Model file for the job. Use its own axes, mm. A direction names the side the tool comes from. Round coordinates to 2 decimals unless told otherwise and drop trailing zeros. Order: outer loops, then holes, each group sorted by start corner. A loop starts at its lowest first (then second) coordinate and runs counter-clockwise, first axis right, second up. Notation, with made-up numbers: (-34.5, 17.5) -> (9.5, 17.5) arc R9 ccw to (9.5, 30.5) -> close; hole circle Ø3 at (-17, 43.25). An arc over 180 degrees is marked (long way). Put each result on its own line as item: value. Start each with the question number.
Q1. 3-axis set-ups, long thin cutter, end or side, ignore diameter. For faces 5 (the face through (-48, 44, 2)), 6 (the face through (30, 44, 2)), 7 (the face through (40, -40, 2)): which of +Z, -Z, +X, -X, +Y, -Y reach the whole face in a straight line?
Q2. Flat gauge pins, fed straight in: P1, Ø1.2, axis at y = -41.5, z = 1, coming from the +X side; P2, Ø1.2, axis at y = -42, z = 2.5, coming from the -X side; P3, Ø2, axis at x = -1, z = 2.5, coming from the +Y side; P4, Ø3, axis at x = 24, y = -5.5, coming from the -Z side. Where does each tip first touch, or does it go through?
Q3. Cut at A-A, the plane y = 41.5. List the corners of the cut face in (x, z).
Q4. Pull direction X, two halves, no side cores. Call faces 1 (the face through (25, 42, 2)), 2 (the face through (-50, 0, 2)), 3 (the face through (-15, -47, 2)), 4 (the face through (-1, 1, 4)): released by +X, released by -X, zero draft, split by the parting line, or undercut.
Q5. Probe L1, parallel to X at y = 41, z = 2.45; L2, parallel to X at y = 49, z = 1; L3, parallel to Y at x = -27, z = 2.3. List the from-to ranges inside material, lowest first.
Q6. Cut at C-C, the plane x = -39.5. List the corners of the cut face in (y, z).
Q7. Cut at B-B, the plane x = 47.5. List the corners of the cut face in (y, z).
from build123d import *

# Parameters (mm, degrees)
SKETCH1_W           = 5
SKETCH1_H           = 4
SKETCH1_W_2         = 4
SKETCH1_H_2         = 10
SKETCH1_W_3         = 10
BOSS_EXTRUDE1_DEPTH = 4
SKETCH2_W           = 4
SKETCH2_H           = 1
BOSS_EXTRUDE2_DEPTH = 4


with BuildPart() as part:
    # Sketch1 → Boss-Extrude1 (new body)
    with BuildSketch(Plane.XY):
        with Locations((-47.5, 42)):
            Rectangle(SKETCH1_W, SKETCH1_H)
        Polygon((-45, 40), (-50, 40), (-50, 35), (-46, 35), (-46, 25), (-50, 25), (-50, 20), (-50, 15), (-46, 15), (-46, 5), (-50, 5), (-50, 0), (-50, -5), (-46, -5), (-46, -15), (-50, -15), (-50, -20), (-50, -25), (-46, -25), (-46, -35), (-50, -35), (-50, -40), (-45, -40), (-40, -40), (-35, -40), (-30, -40), (-25, -40), (-20, -40), (-15, -40), (-10, -40), (-5, -40), (0, -40), (5, -40), (10, -40), (15, -40), (20, -40), (25, -40), (30, -40), (35, -40), (40, -40), (45, -40), (50, -40), (50, -35), (46, -35), (46, -25), (50, -25), (50, -20), (50, -15), (46, -15), (46, -5), (50, -5), (50, 0), (50, 5), (46, 5), (46, 15), (50, 15), (50, 20), (50, 25), (46, 25), (46, 35), (50, 35), (50, 40), (45, 40), (40, 40), (35, 40), (30, 40), (25, 40), (20, 40), (15, 40), (10, 40), (5, 40), (0, 40), (-5, 40), (-10, 40), (-15, 40), (-20, 40), (-25, 40), (-30, 40), (-35, 40), (-40, 40), align=None)
        with Locations((-48, 30)):
            Rectangle(SKETCH1_W_2, SKETCH1_H_2)
        with Locations((-52, 30)):
            Rectangle(SKETCH1_W_2, SKETCH1_H_2)
        Polygon((-35, 44), (-35, 40), (-30, 40), (-25, 40), (-25, 44), align=None)
        with Locations((-48, 10)):
            Rectangle(SKETCH1_W_2, SKETCH1_H_2)
        with Locations((-52, 10)):
            Rectangle(SKETCH1_W_2, SKETCH1_H_2)
        Polygon((-15, 44), (-15, 40), (-10, 40), (-5, 40), (-5, 44), align=None)
        with Locations((-48, -10)):
            Rectangle(SKETCH1_W_2, SKETCH1_H_2)
        with Locations((-52, -10)):
            Rectangle(SKETCH1_W_2, SKETCH1_H_2)
        with Locations((-10, 49)):
            Rectangle(SKETCH1_W_3, SKETCH1_H_2)
        with Locations((-48, -30)):
            Rectangle(SKETCH1_W_2, SKETCH1_H_2)
        with Locations((-52, -30)):
            Rectangle(SKETCH1_W_2, SKETCH1_H_2)
        Polygon((5, 44), (5, 40), (10, 40), (15, 40), (15, 44), align=None)
        with Locations((10, 49)):
            Rectangle(SKETCH1_W_3, SKETCH1_H_2)
        with Locations((-47.5, -42)):
            Rectangle(SKETCH1_W, SKETCH1_H)
        Polygon((25, 44), (25, 40), (30, 40), (35, 40), (35, 44), align=None)
        Polygon((-30, -40), (-35, -40), (-35, -44), (-25, -44), (-25, -40), align=None)
        with Locations((47.5, 42)):
            Rectangle(SKETCH1_W, SKETCH1_H)
        Polygon((-10, -40), (-15, -40), (-15, -44), (-5, -44), (-5, -40), align=None)
        with Locations((-10, -49)):
            Rectangle(SKETCH1_W_3, SKETCH1_H_2)
        with Locations((52, 30)):
            Rectangle(SKETCH1_W_2, SKETCH1_H_2)
        with Locations((48, 30)):
            Rectangle(SKETCH1_W_2, SKETCH1_H_2)
        Polygon((10, -40), (5, -40), (5, -44), (15, -44), (15, -40), align=None)
        with Locations((52, 10)):
            Rectangle(SKETCH1_W_2, SKETCH1_H_2)
        with Locations((48, 10)):
            Rectangle(SKETCH1_W_2, SKETCH1_H_2)
        with Locations((10, -49)):
            Rectangle(SKETCH1_W_3, SKETCH1_H_2)
        with Locations((52, -10)):
            Rectangle(SKETCH1_W_2, SKETCH1_H_2)
        with Locations((48, -10)):
            Rectangle(SKETCH1_W_2, SKETCH1_H_2)
        Polygon((30, -40), (25, -40), (25, -44), (35, -44), (35, -40), align=None)
        with Locations((52, -30)):
            Rectangle(SKETCH1_W_2, SKETCH1_H_2)
        with Locations((48, -30)):
            Rectangle(SKETCH1_W_2, SKETCH1_H_2)
        with Locations((47.5, -42)):
            Rectangle(SKETCH1_W, SKETCH1_H)
    extrude(amount=BOSS_EXTRUDE1_DEPTH)

    # Sketch2 → Boss-Extrude2 (add)
    with BuildSketch(Plane.XY.offset(4)):
        with Locations((52, -35.5)):
            Rectangle(SKETCH2_W, SKETCH2_H)
        with Locations((52, 35.5)):
            Rectangle(SKETCH2_W, SKETCH2_H)
        with Locations((-52, -35.5)):
            Rectangle(SKETCH2_W, SKETCH2_H)
        with Locations((-52, 35.5)):
            Rectangle(SKETCH2_W, SKETCH2_H)
    extrude(amount=-BOSS_EXTRUDE2_DEPTH)


solid = part.part
Ans:
1. face 5: +Z, -Z, -X, +Y
1. face 6: +Z, -Z, +X, +Y
1. face 7: +Z, -Z, -Y
2. P1: stops at x = 50
2. P2: stops at x = -50
2. P3: stops at y = 40
2. P4: stops at z = 0
3. outline: (-50, 0) -> (-45, 0) -> (-45, 4) -> (-50, 4) -> close; (-35, 0) -> (-25, 0) -> (-25, 4) -> (-35, 4) -> close; (-15, 0) -> (-5, 0) -> (-5, 4) -> (-15, 4) -> close; (5, 0) -> (15, 0) -> (15, 4) -> (5, 4) -> close; (25, 0) -> (35, 0) -> (35, 4) -> (25, 4) -> close; (45, 0) -> (50, 0) -> (50, 4) -> (45, 4) -> close
4. face 1: undercut
4. face 2: released by -X
4. face 3: undercut
4. face 4: zero draft
5. L1: x = -50 to -45, -35 to -25, -15 to -5, 5 to 15, 25 to 35, 45 to 50
5. L2: x = -15 to -5, 5 to 15
5. L3: y = -44 to 44
6. outline: (-40, 0) -> (40, 0) -> (40, 4) -> (-40, 4) -> close
7. outline: (-44, 0) -> (44, 0) -> (44, 4) -> (-44, 4) -> close
